Check sheet for the modelled part. Datum: model origin and axes. Units: mm. Face numbers are marked on the shaded views. A direction names the side the tool comes from. Round coordinates to 2 decimals unless told otherwise and drop trailing zeros. Write each loop counter-clockwise with the first axis right and the second up, starting at its lowest first coordinate (ties: lowest second). Pieces come first, ordered by that corner, then holes. Notation, with made-up numbers: M -15.5,-1 L -5.5,-1 A17 cw -5.5,8 Z; hole C 14,-24 d10. An arc over 180 degrees is marked long. One line per item, written item: value.
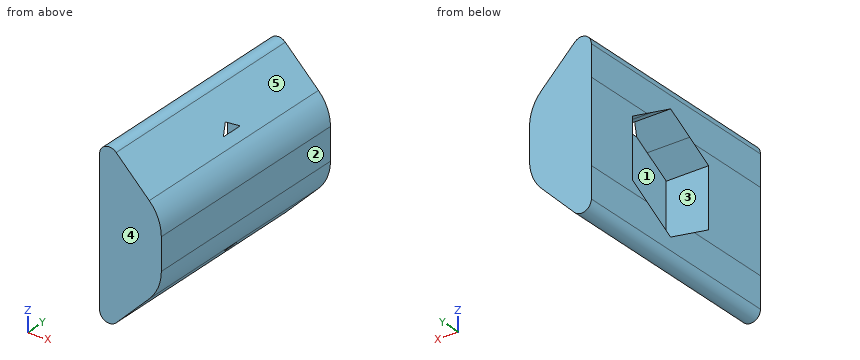
from build123d import *

# Parameters (mm, degrees)
BOSS_EXTRUDE1_START = 3
BOSS_EXTRUDE1_DEPTH = 8
CUT_EXTRUDE1_DEPTH  = 3


with BuildPart() as part:
    # Sketch1 → Boss-Extrude1 (new, symmetric)
    with BuildSketch(Plane(origin=(0, 887.368143731, 0), x_dir=(1, 0, 0), z_dir=(0, 1, 0)).offset(BOSS_EXTRUDE1_START)):
        with BuildLine():
            Line((637.813700875, -1272.18749392), (637.81370087, -1269.938359702))
            ThreePointArc((637.81370087, -1269.938359702), (637.592190309, -1268.824750917), (636.961381603, -1267.880678974))
            Line((636.961381603, -1267.880678974), (634.621604573, -1265.540901944))
            ThreePointArc((634.621604573, -1265.540901944), (633.86964944, -1265.391328698), (633.443700894, -1266.028805374))
            Line((633.443700894, -1266.028805374), (633.443700112, -1268.19792696))
            Line((633.443700112, -1268.19792696), (633.443700112, -1273.927926678))
            Line((633.443700112, -1273.927926678), (633.4437009, -1276.09704826))
            ThreePointArc((633.4437009, -1276.09704826), (633.869649447, -1276.734524935), (634.621604579, -1276.584951689))
            Line((634.621604579, -1276.584951689), (636.961381608, -1274.245174659))
            ThreePointArc((636.961381608, -1274.245174659), (637.592190316, -1273.301102712), (637.813700875, -1272.18749392))
        make_face()
    extrude(amount=BOSS_EXTRUDE1_DEPTH, both=True)

    # Sketch2 → Cut-Extrude1 (cut)
    with BuildSketch(Plane(origin=(633.443237581, 0, -0.000229987), x_dir=(3.630749913810974e-07, 0, 0.9999999999999342), z_dir=(-0.9999999999999342, 0, 3.630749913810974e-07))):
        Polygon((1268.987365094, 887.268143731), (1267.948134548, 889.068143719), (1266.908904124, 890.868143731), (1267.948134534, 892.668143718), (1268.987365094, 894.468143731), (1271.065825986, 894.468143731), (1273.144287032, 894.468143731), (1274.18351745, 892.668143728), (1275.222748001, 890.868143731), (1274.183517448, 889.068143728), (1273.144287032, 887.268143731), (1271.065825995, 887.268143731), align=None)
    extrude(amount=-CUT_EXTRUDE1_DEPTH, mode=Mode.SUBTRACT)


solid = part.part
Q1. Sectioned sample at A-A on x = 634.25. Enter the section's corners in (y, z).
Completed:
outline: M 882.37,1265.35 L 898.37,1265.35 L 898.37,1276.78 L 882.37,1276.78 Z; hole M 887.27,1268.99 L 890.87,1266.91 L 894.47,1268.99 L 894.47,1273.14 L 890.87,1275.22 L 887.27,1273.14 Z
Q2. Scan lines: line 1 (X direction, y = 893.75, z = 1271.75); line 2 (Y direction, x = 633.95, z = 1268.75); line 3 (Z direction, x = 634.1, y = 891.5). Record each from-to range of solid material in increasing order. Write a range as [from, to].
Completed:
line 1: [636.44, 637.81]
line 2: [882.37, 887.68], [894.06, 898.37]
line 3: [1265.34, 1267.27], [1274.86, 1276.79]
Q3. Access from +Z, -Z, +X, -X, +Y, -Y to the whole of each face (thin tool, end or side, straight path). Record for the marked faces 1 and 2.
Completed:
face 1: -X
face 2: +Z, -Z, +X, +Y, -Y
Q4. Sectioned sample at C-C on z = 1271.5. Enter the section's corners in (x, y), and give its area (3 significant figures).
Completed:
outline: M 633.44,882.37 L 637.81,882.37 L 637.81,898.37 L 633.44,898.37 L 633.44,894.47 L 636.44,894.47 L 636.44,887.27 L 633.44,887.27 Z
area: 48.3 mm^2
Q5. Depth check by flat-ended pin: P1, Ø2, axis at y = 892.5, z = 1270, coming from the -X side. Enter the tip coordinate at first touch or a pass-through.
Completed:
P1: x = 636.44
Q6. Draft check along Z on the marked faces 3, 4 and 5. Enter one of: pulls with the +Z half, pulls with the -Z half, needs draft (parallel to the pull), parting line crosses it, or undercut.
Completed:
face 3: undercut
face 4: needs draft
face 5: pulls with the +Z half
Q7. Sectioned sample at B-B on y = 896.25. Enter the section's corners in (x, z), and give its area (3 significant figures).
Completed:
outline: M 633.44,1266.03 A0.69 ccw 634.62,1265.54 L 636.96,1267.88 A2.91 ccw 637.81,1269.94 L 637.81,1272.19 A2.91 ccw 636.96,1274.25 L 634.62,1276.58 A0.69 ccw 633.44,1276.1 L 633.44,1273.93 L 633.44,1268.2 Z
area: 37.9 mm^2
Q8. Sectioned sample at D-D on x = 637.3. Enter the section's corners in (y, z).
Completed:
outline: M 882.37,1268.29 L 898.37,1268.29 L 898.37,1273.84 L 882.37,1273.84 Z
